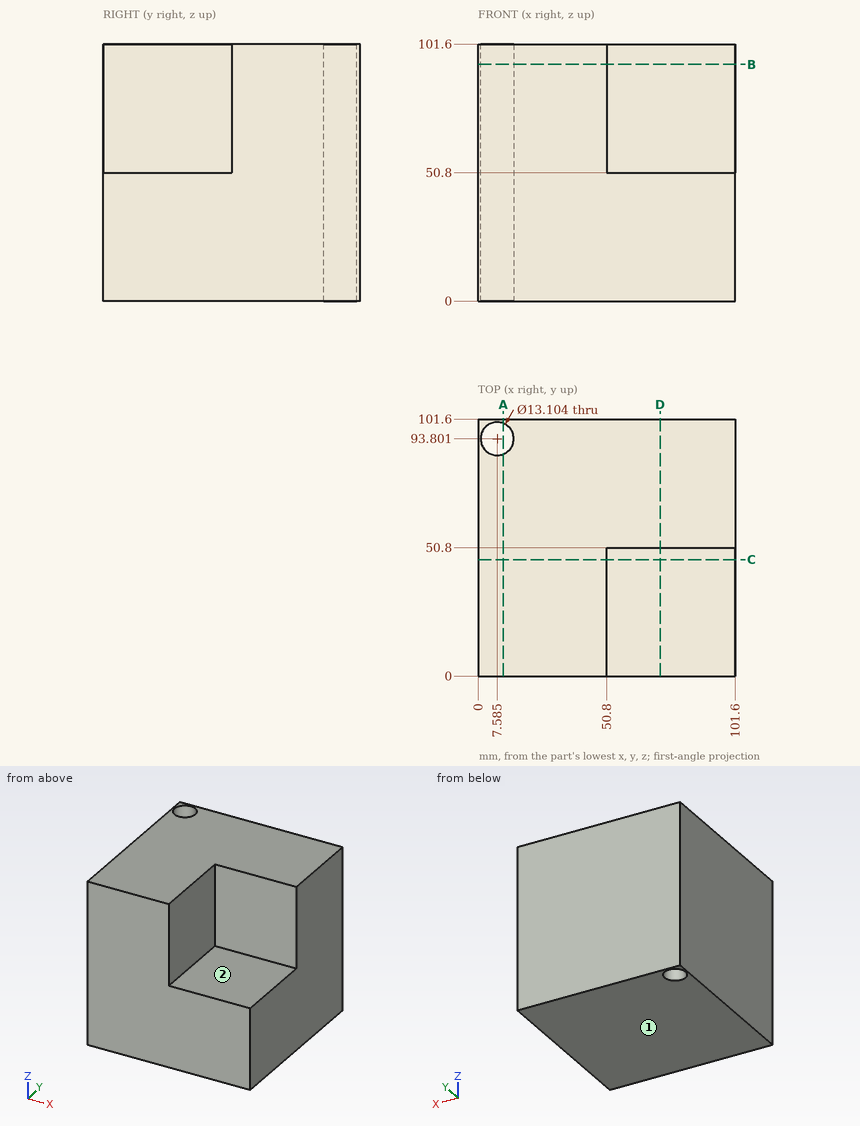
Can you work these out from the drawing? Everything is in mm from the part's minimum corner. A direction names the side the tool comes from. Give positions to 0.01 mm unless a question says otherwise; leave off trailing zeros. Order: outer loops, then holes, each group sorted by start corner. A loop starts at its lowest first (then second) coordinate and runs counter-clockwise, first axis right, second up. Notation, with made-up numbers: M -16.5,84.25 L 11.5,84.25 A33 cw 11.5,117.25 Z; hole C -29.75,82 d3. An arc over 180 degrees is marked long. One line per question, with ' | ' between items.
1. I want a section at C-C (y = 46). List the corners of the cut face in (x, z) for me, and give its area (3 significant figures).
Results:
outline: M 0,0 L 101.6,0 L 101.6,50.8 L 50.8,50.8 L 50.8,101.6 L 0,101.6 Z | area: 7,740 mm²
2. I want a section at A-A (x = 10). List the corners of the cut face in (y, z) for me.
Results:
outline: M 0,0 L 87.71,0 L 87.71,101.6 L 0,101.6 Z; M 99.89,0 L 101.6,0 L 101.6,101.6 L 99.89,101.6 Z
3. I want a section at B-B (z = 93.5). List the corners of the cut face in (x, y) for me (1 decimal), and give its area (3 significant figures).
Results:
outline: M 0,0 L 50.8,0 L 50.8,50.8 L 101.6,50.8 L 101.6,101.6 L 0,101.6 Z; hole C 7.6,93.8 d13.1 | area: 7,610 mm²
4. I'm going to push flat-ended pins straight in: pin 1 (8 mm diameter, centred on x = 75.5, z = 81.5, fed in from -Y); pin 2 (10.5 mm diameter, centred on x = 7.59, y = 93.8, fed in from +Z). Where does each tip first touch, or does it pass through?
Results:
pin 1: y = 50.8 | pin 2: through
5. I want a section at D-D (x = 72). List the corners of the cut face in (y, z) for me.
Results:
outline: M 0,0 L 101.6,0 L 101.6,101.6 L 50.8,101.6 L 50.8,50.8 L 0,50.8 Z
6. For the marked faces 1 and 2, which set-ups out of +Z, -Z, +X, -X, +Y, -Y let a thin tool reach every point of the face, with its end or its side?
Results:
face 1: -Z, +X, -X, +Y, -Y | face 2: +Z, +X, -Y
7. If I drill on line 1 (Y direction, x = 8, z = 38); line 2 (Z direction, x = 96.5, y = 41.5); line 3 (Y direction, x = 66, z = 94), over which ranges is the centre line in solid material (lowest first)?
Results:
line 1: 0 to 87.26, 100.34 to 101.6 | line 2: 0 to 50.8 | line 3: 50.8 to 101.6
